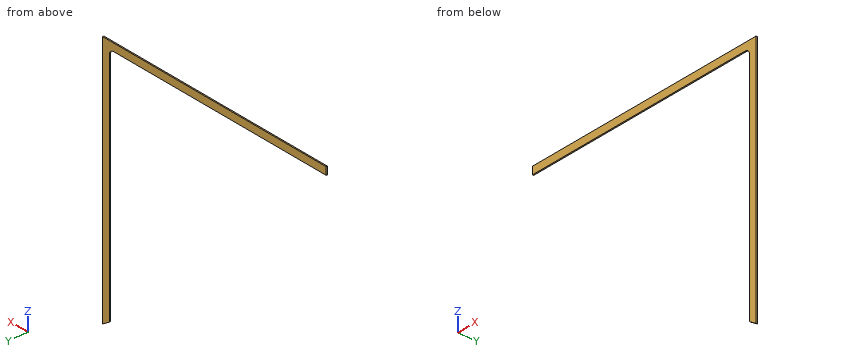
from build123d import *

# Parameters (mm, degrees)
BOSS_EXTRUDE2_DEPTH = 0.125
FILLET2_R           = 1


with BuildPart() as part:
    # Sketch2 → Boss-Extrude2 (new, symmetric)
    with BuildSketch(Plane(origin=(0, 0, 0), x_dir=(1, 0, 0), z_dir=(0, 1, 0))):
        Polygon((0, 0), (0, 47.5), (1.5, 48.5), (1.5, -1.5), (-48.5, -1.5), (-48.5, 0), align=None)
    extrude(amount=BOSS_EXTRUDE2_DEPTH, both=True)

    # Fillet2
    fillet2_edges = [part.edges().sort_by_distance(p)[0] for p in [
        (0, 0, 0),
    ]]
    fillet(fillet2_edges, radius=FILLET2_R)


solid = part.part
The model under review builds one solid part; all positions refer to its coordinate system, in mm. Round coordinates to 2 decimals unless told otherwise and drop trailing zeros. Loops run counter-clockwise (first coordinate to the right, second up) from the corner with the lowest first, then second, coordinate; pieces in that order, holes last. Notation, with made-up numbers: (-16, 55) -> (21, 55) arc R29 ccw to (21, 77) -> close; hole circle Ø10 at (88.5, -29). An arc over 180 degrees is marked (long way). Return JSON: item names as keys, results as strings.
(1) Add section C-C on z = -32. Write out the cut boundary in (x, y) (3 decimals), plus the area to 3 significant figures.
Solved:
{"outline": "(0, -0.125) -> (1.5, -0.125) -> (1.5, 0.125) -> (0, 0.125) -> close", "area": "0.375 mm2"}
(2) Add section A-A on y = 0. Write out the cut boundary in (x, z).
Solved:
{"outline": "(-48.5, 0) -> (-1, 0) arc R1 cw to (0, -1) -> (0, -47.5) -> (1.5, -48.5) -> (1.5, 1.5) -> (-48.5, 1.5) -> close"}
(3) For line 1 (X direction, y = -0.05, z = -20.5), list the stretches that pass through material, from the lowest coordinate up.
Solved:
{"line 1": "0 to 1.5"}
(4) Add section B-B on x = -45. Write out the cut boundary in (y, z) (3 decimals).
Solved:
{"outline": "(-0.125, 0) -> (0.125, 0) -> (0.125, 1.5) -> (-0.125, 1.5) -> close"}
